The listing builds one solid part. Answer for the finished solid, in the listing's coordinates (mm). A direction names the side the tool comes from. Round coordinates to 2 decimals unless told otherwise and drop trailing zeros. Order: outer loops, then holes, each group sorted by start corner. A loop starts at its lowest first (then second) coordinate and runs counter-clockwise, first axis right, second up. Notation, with made-up numbers: (52, 33) - (59, 33) arc R3 cw to (59, 37) - close; hole circle Ø4 at (72.25, 8). An arc over 180 degrees is marked (long way). One line per item, written item: value. Start each with the question number.
1. Section B-B, the plane x = 0 is taken. Give the vertices of the cut face in (y, z) (3 decimals).
2. A tool of negligible diameter and unlimited length cuts with its end or side. For faces 1 (the flat face through (-5, 22, 14)), 2 (the cylindrical face through (-5.52, 11.15, 13.3)), from which of +Z, -Z, +X, -X, +Y, -Y can it reach the whole face along a straight path? Write none if from no direction.
3. Section D-D, the plane z = 9.5 is taken. Give the vertices of the cut face in (x, y), then the cut area to 3 significant figures.
4. Section C-C, the plane y = 18.25 is taken. Give the vertices of the cut face in (x, z).
5. Section A-A, the plane z = -5 is taken. Give the vertices of the cut face in (x, y), then the cut area to 3 significant figures.
6. Flat-ended cylindrical pins translate along their axes: P1, Ø4.5, axis at x = 1.5, z = 1, coming from the +Y side; P2, Ø6, axis at y = 9.5, z = 6.5, coming from the +X side; P3, Ø1.5, axis at x = 2, z = 6, coming from the +Y side; P4, Ø1.2, axis at x = -2.71, z = 5.35, coming from the -Y side. Find the tip coordinate at first contact, or state that the pin passes through.
7. Straight lines are drawn through the part: line 1 (Y direction, x = -6, z = -9); line 2 (X direction, y = 6.5, z = 0); line 3 (X direction, y = -0.25, z = 0) (3 decimals). For each, find the intervals that lie inside material, in ascending order.
8. For a pull along X with two mould halves and no side action, classify faces 3 (the flat face through (0, -3, 0)), 4 (the cylindrical face through (-9.49, 9.68, -12.38)), 5 (the cylindrical face through (5.015, -1.521, -0.11)) as released by +X, released by -X, zero draft, split by the parting line, or undercut.
from build123d import *

# Parameters (mm, degrees)
SKETCH1_R           = 15.6
BOSS_EXTRUDE1_DEPTH = 3
SKETCH2_R           = 4.275
CUT_EXTRUDE1_DEPTH  = 1.5
BOSS_EXTRUDE2_START = 22
SKETCH3_R           = 15.6
SKETCH3_R_2         = 14.4
BOSS_EXTRUDE2_DEPTH = 22
SKETCH4_R           = 1
CUT_EXTRUDE3_DEPTH  = 3


with BuildPart() as part:
    # Sketch1 → Boss-Extrude1 (new body)
    with BuildSketch(Plane(origin=(0, 0, 0), x_dir=(1, 0, 0), z_dir=(0, 1, 0))):
        with Locations(Location((0, 0, 0), (0, 0, 270))):
            Circle(SKETCH1_R)
    extrude(amount=-BOSS_EXTRUDE1_DEPTH)

    # Sketch2 → Cut-Extrude1 (cut)
    with BuildSketch(Plane(origin=(0, 0, 0), x_dir=(1, 0, 0), z_dir=(0, 1, 0))):
        with Locations(Location((0, 0, 0), (0, 0, 270))):
            Circle(SKETCH2_R)
    extrude(amount=-CUT_EXTRUDE1_DEPTH, mode=Mode.SUBTRACT)

    # Sketch3 → Boss-Extrude2 (add)
    with BuildSketch(Plane(origin=(0, 0, 0), x_dir=(1, 0, 0), z_dir=(0, 1, 0)).offset(BOSS_EXTRUDE2_START)):
        with Locations(Location((0, 0, 0), (0, 0, 270))):
            Circle(SKETCH3_R)
        with Locations(Location((0, 0, 0), (0, 0, 270))):
            Circle(SKETCH3_R_2, mode=Mode.SUBTRACT)
    extrude(amount=-BOSS_EXTRUDE2_DEPTH)

    # Sketch4 → Cut-Extrude3 (cut)
    with BuildSketch(Plane(origin=(0, -3, 0), x_dir=(-1, 0, 0), z_dir=(0, -1, 0))):
        with Locations(Location((-5.991069688, 0.327236899, 0), (0, 0, 90))):
            Circle(SKETCH4_R)
        with Locations(Location((3.278930312, 5.024800097, 0), (0, 0, 270))):
            Circle(SKETCH4_R)
        with Locations(Location((2.712139377, -5.352036995, 0), (0, 0, 270))):
            Circle(SKETCH4_R)
    extrude(amount=-CUT_EXTRUDE3_DEPTH, mode=Mode.SUBTRACT)


solid = part.part
Answer list:
1. outline: (-3, -15.6) - (22, -15.6) - (22, -14.4) - (0, -14.4) - (0, -4.275) - (-1.5, -4.275) - (-1.5, 4.275) - (0, 4.275) - (0, 14.4) - (22, 14.4) - (22, 15.6) - (-3, 15.6) - close
2. face 1: +Z, -Z, +X, -X, +Y
2. face 2: +Y
3. outline: (-12.37, -3) - (12.37, -3) - (12.37, 22) - (10.82, 22) - (10.82, 0) - (-10.82, 0) - (-10.82, 22) - (-12.37, 22) - close
3. area: 143 mm²
4. outline: circle Ø31.2 at (0, 0); hole circle Ø28.8 at (0, 0)
5. outline: (-14.78, -3) - (-4.28, -3) - (-4.28, 0) - (-13.5, 0) - (-13.5, 22) - (-14.78, 22) - close; (-2.28, -3) - (14.78, -3) - (14.78, 22) - (13.5, 22) - (13.5, 0) - (-2.28, 0) - close
5. area: 139 mm²
6. P1: stops at y = -1.5
6. P2: stops at x = 15.2
6. P3: stops at y = 0
6. P4: passes through
7. line 1: y = -3 to 0
7. line 2: x = -15.6 to -14.4, 14.4 to 15.6
7. line 3: x = -15.6 to -4.275, 4.275 to 5.046, 6.936 to 15.6
8. face 3: zero draft
8. face 4: split by the parting line
8. face 5: undercut
